Autodesk Inventor part; units mm, degrees
ref_plane "Work Plane1" through (-7.5007, -7.5, 224.8016) normal (0, 0, -1) x (0, 1, 0)
ref_plane "YZ Plane" through (0, 0, 0) normal (1, 0, 0) x (0, 1, 0)
ref_plane "XZ Plane" through (0, 0, 0) normal (0, 1, 0) x (-1, 0, 0)
sketch "Sketch1" plane through (0, 0, 0) normal (0, 0, 1) x (1, 0, 0)
  circle A0 centre (-0.0005, 100.4366) radius 2.5
  arc A1 (7.4995, 100.4366) -> (-7.5005, 100.4366) centre (-0.0005, 100.4366) ccw
  circle A2 centre (-0.0005, 100.4366) radius 7.5
  arc A3 (11.4995, 100.4366) -> (-11.5005, 100.4365) centre (-0.0005, 100.4366) ccw
  circle A4 centre (-0.0005, 100.4366) radius 11.5
  line L0 (-0.0005, 100.4366) -> (11.4995, 107.0761)
  line L1 (-0.0005, 100.4366) -> (16.6776, 100.4366) construction
  line L2 (-0.0005, 111.9366) -> (9.9588, 106.1866)
  line L3 (5.7495, 110.3959) -> (4.9792, 109.0616)
  line L4 (-0.0005, 113.7156) -> (11.4995, 107.0761)
  line L5 (-4.6563, 116.4037) -> (19.5852, 116.4037) construction
  line L6 (-0.0005, 100.4366) -> (-0.0005, 113.7156)
  line L7 (-11.5005, 107.0761) -> (-0.0005, 113.7156)
  line L8 (-11.5005, 93.7971) -> (-11.5005, 107.0761)
  line L9 (-0.0005, 87.1575) -> (-11.5005, 93.7971)
  line L10 (11.4995, 93.7971) -> (-0.0005, 87.1575)
  line L11 (11.4995, 107.0761) -> (11.4995, 93.7971)
  point P0 (0, 0)
  point P1 (11.4995, 100.4366)
  point P2 (11.4995, 100.4366)
  dimension "d0" = 30
  dimension "d1" = 30
  dimension "d4" = 360
ref_plane "Work Plane1" through (-7.5007, -7.5, 224.8016) normal (0, 0, -1) x (0, 1, 0)
extrude "Extrusion1" add sketch "Sketch1" along normal up to surface (224.8016 mm away) contours A0 L0 A1 A2 L6 | A0 L6 A1 L0 | L0 A3 A4 L6 A1 A2 | A1 L6 L2 L0 | L0 L11 A3 | L2 L3 A3 | A3 L4 L0 | L6 L4 A3 | A3 L3 L2 | A3 L7 L6 | L11 L10 A4 | A3 L8 L7 | L10 L9 A4 | A4 L9 L8
properties part number "TheHandleBar_3DPrint"
Check sheet for the modelled part. Datum: model origin and axes. Units: mm. Coordinates: 2 decimals unless noted, no trailing zeros. Write each loop counter-clockwise with the first axis right and the second up, starting at its lowest first coordinate (ties: lowest second). Pieces come first, ordered by that corner, then holes. Notation, with made-up numbers: (51, -9.75) - (63, -9.75) arc R12 ccw to (63, 13.25) - close; hole circle Ø7 at (-12, -13). An arc over 180 degrees is marked (long way). One line per question, with ' | ' between items.
Item 1: Sectioned sample at C-C on x = -4.75. Record the boundary of the cut face in (y, z).
Determined:
outline: (89.9, 0) - (110.97, 0) - (110.97, 224.8) - (89.9, 224.8) - close
Item 2: Sectioned sample at B-B on y = 91. Record the boundary of the cut face in (x, z).
Determined:
outline: (-6.66, 0) - (6.65, 0) - (6.65, 224.8) - (-6.66, 224.8) - close
Item 3: Sectioned sample at A-A on z = 90.5. Record the boundary of the cut face in (x, y).
Determined:
outline: (-11.5, 93.8) - (0, 87.16) - (11.5, 93.8) - (11.5, 107.08) - (0, 113.72) - (-11.5, 107.08) - close; hole circle Ø5 at (0, 100.44)
Item 4: Gauge pin test, flat ends, axial feed: P1, Ø10, axis at x = -6, z = 180, coming from the +Y side; P2, Ø8, axis at x = -5.5, z = 139, coming from the +Y side; P3, Ø4, axis at y = 90, z = 73.5, coming from the -X side. Record the tip position at first contact, or that the pin passes through.
Determined:
P1: stops at y = 113.14 | P2: stops at y = 112.85 | P3: stops at x = -8.39
Item 5: Mould release check, pull along Y, two halves, no side actions. Record for faces 1 (the face through (-0.542, 102.877, 110.827)), 2 (the face through (-0.2, 97.7, 0)), 3 (the face through (-5.83, 110.35, 110.83)): pulls with the +Y half, pulls with the -Y half, needs draft (parallel to the pull), parting line crosses it, or undercut.
Determined:
face 1: undercut | face 2: needs draft | face 3: pulls with the +Y half
Item 6: Thickness scan on line 1 (Y direction, x = -2.25, z = 175); line 2 (Y direction, x = -0.5, z = 10.5); line 3 (X direction, y = 101, z = 40.5). Record the ranges inside material, lowest first. Write a range as [from, to].
Determined:
line 1: y = [88.46, 99.35], [101.53, 112.42] | line 2: y = [87.45, 97.99], [102.89, 113.43] | line 3: x = [-11.5, -2.44], [2.44, 11.5]
